For this review, use the dimensioned drawing (mm, ordinates from the lowest corner) and the shaded views. A direction names the side the tool comes from. Give positions to 0.01 mm unless a question says otherwise; leave off trailing zeros. Write each loop counter-clockwise with the first axis right and the second up, starting at its lowest first coordinate (ties: lowest second). Pieces come first, ordered by that corner, then holes. Notation, with made-up numbers: (-28, 3.5) -> (-1, 3.5) arc R13 cw to (-1, 18.5) -> close; hole circle Ø9 at (30.25, 82). An arc over 180 degrees is marked (long way). Return JSON: item names as keys, results as strings.
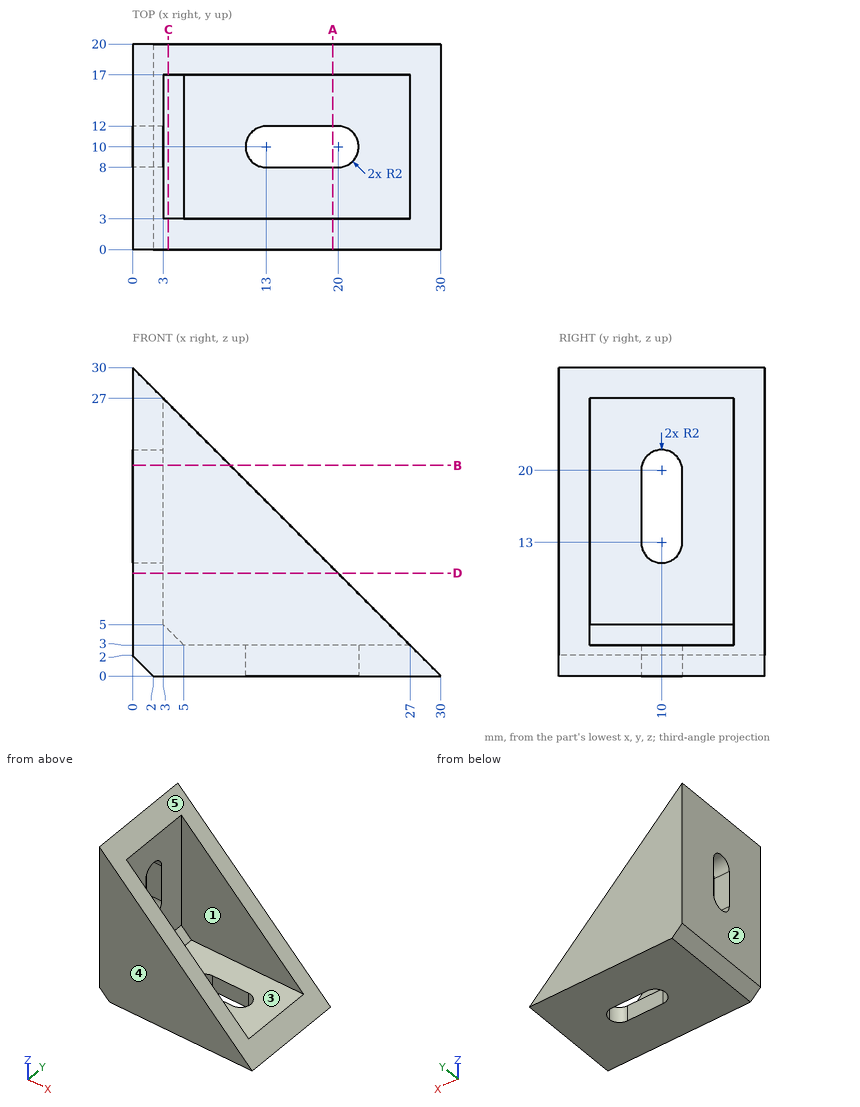
1. Add section C-C, the plane x = 3.5. State the section outline as (y, z) points.
Results found:
{"outline": "(0, 0) -> (20, 0) -> (20, 26.5) -> (17, 26.5) -> (17, 4.5) -> (3, 4.5) -> (3, 26.5) -> (0, 26.5) -> close"}
2. Add section A-A, the plane x = 19.5. State the section outline as (y, z) points.
Results found:
{"outline": "(0, 0) -> (8, 0) -> (8, 3) -> (3, 3) -> (3, 10.5) -> (0, 10.5) -> close; (12, 0) -> (20, 0) -> (20, 10.5) -> (17, 10.5) -> (17, 3) -> (12, 3) -> close"}
3. Add section B-B, the plane z = 20.5. State the section outline as (x, y) points, plus the area to 3 significant figures.
Results found:
{"outline": "(0, 0) -> (9.5, 0) -> (9.5, 3) -> (3, 3) -> (3, 8.06) -> (0, 8.06) -> close; (0, 11.94) -> (3, 11.94) -> (3, 17) -> (9.5, 17) -> (9.5, 20) -> (0, 20) -> close", "area": "87.4 mm²"}
4. For pin 1 (4 mm diameter, centred on x = 25, y = 16.5, fed in from +Z); pin 2 (4 mm diameter, centred on x = 18.5, y = 8.5, fed in from +Z); pin 3 (7 mm diameter, centred on x = 17.5, z = 18, fed in from -Y), all flat-tipped, find the tip position at first contact; note any pin that passes through.
Results found:
{"pin 1": "stops at z = 6.94", "pin 2": "stops at z = 3", "pin 3": "passes through"}
5. For the marked faces 1 and 2, list the 3-axis set-ups (+Z, -Z, +X, -X, +Y, -Y) from which the entire face can be reached by the end or side of a thin tool; tool diameter is ignored.
Results found:
{"face 1": "+Z, +X", "face 2": "+Z, -Z, -X, +Y, -Y"}
6. Add section D-D, the plane z = 10. State the section outline as (x, y) points, plus the area to 3 significant figures.
Results found:
{"outline": "(0, 0) -> (20, 0) -> (20, 3) -> (3, 3) -> (3, 17) -> (20, 17) -> (20, 20) -> (0, 20) -> close", "area": "162 mm²"}
7. The part is to be moulded in two halves that separate along Y. For the marked faces 3, 4 and 5, say which applies: +Y half, -Y half, draft (parallel to the pull), parting line (faces both ways), or undercut.
Results found:
{"face 3": "undercut", "face 4": "-Y half", "face 5": "draft"}
8. To check wall thickness, follow probe 1 along Z at (x, y) = (10, 14.25); probe 2 along Y at (x, z) = (7, 11). State the ranges of each line that lie inside material, in increasing order.
Results found:
{"probe 1": "z = 0 to 3", "probe 2": "y = 0 to 3, 17 to 20"}
